from build123d import *

# Parameters (mm, degrees)
BOSS_EXTRUDE1_DEPTH = 9
SKETCH2_R           = 2.5
CUT_EXTRUDE1_DEPTH  = 39.913365313
BOSS_EXTRUDE2_DEPTH = 4.5
CUT_EXTRUDE2_DEPTH  = 3.5


with BuildPart() as part:
    # Sketch1 → Boss-Extrude1 (new body)
    with BuildSketch(Plane.XY):
        with BuildLine():
            Line((0, 0), (0, -5.580710666))
            ThreePointArc((0, -5.580710666), (0.901780583, -8.110737631), (3.200518222, -9.5))
            Line((3.200518222, -9.5), (13.019339267, -11.502906099))
            ThreePointArc((13.019339267, -11.502906099), (17.074073947, -15.986411077), (14, -21.191481642))
            Line((14, -21.191481642), (14, -31.5))
            Line((14, -31.5), (21, -31.5))
            Line((21, -31.5), (21, -5.5))
            Line((21, -5.5), (4, -5.5))
            Line((4, -5.5), (4, 0))
            Line((4, 0), (0, 0))
        make_face()
    extrude(amount=BOSS_EXTRUDE1_DEPTH)

    # Sketch2 → Cut-Extrude1 (cut, through all)
    with BuildSketch(Plane(origin=(21, 0, 0), x_dir=(0, 0, -1), z_dir=(1, 0, 0))):
        with Locations((-6, -25.5)):
            Circle(SKETCH2_R)
    extrude(amount=-CUT_EXTRUDE1_DEPTH, mode=Mode.SUBTRACT)

    # Sketch3 → Boss-Extrude2 (add)
    with BuildSketch(Plane.XY.offset(9)):
        with BuildLine():
            Line((12, -5.5), (12, -11.294974737))
            Line((12, -11.294974737), (13.019339267, -11.502906099))
            ThreePointArc((13.019339267, -11.502906099), (17.074073947, -15.986411077), (14, -21.191481642))
            Line((14, -21.191481642), (14, -31.5))
            Line((14, -31.5), (21, -31.5))
            Line((21, -31.5), (21, -5.5))
            Line((21, -5.5), (12, -5.5))
        make_face()
    extrude(amount=BOSS_EXTRUDE2_DEPTH)

    # Sketch4 → Cut-Extrude2 (cut)
    with BuildSketch(Plane(origin=(21, 0, 0), x_dir=(0, 0, -1), z_dir=(1, 0, 0))):
        Polygon((-10.2, -23.652479139), (-10.2, -27.347520861), (-6, -29.772391992), (-2.3, -27.636195996), (-2.3, -23.363804004), (-6, -21.227608008), align=None)
    extrude(amount=-CUT_EXTRUDE2_DEPTH, mode=Mode.SUBTRACT)


solid = part.part
Check sheet for the modelled part. Datum: model origin and axes. Units: mm. A direction names the side the tool comes from. Give positions to 0.01 mm unless a question says otherwise; leave off trailing zeros. Loops run counter-clockwise (first coordinate to the right, second up) from the corner with the lowest first, then second, coordinate; pieces in that order, holes last. Notation, with made-up numbers: M 27,11 L 44,11 A6 cw 44,17 Z; hole C 67.5,14.5 d3. An arc over 180 degrees is marked long. Use a Markdown table: item, result. Add a question column.
Q1. Sectioned sample at B-B, the plane x = 15. Record the cut outline in (y, z).
Q2. Scan lines: line 1 along Y through (x, z) = (15.1, 6); line 2 along X through (y, z) = (-28, 1.75); line 3 along X through (y, z) = (-10, 11). Record each from-to range of solid material in increasing order. Write a range as [from, to].
Q3. Sectioned sample at A-A, the plane y = -25.5. Record the cut outline in (x, z).
Q4. Mould release check, pull along Y, two halves, no side actions. Record for faces 5 (the flat face through (17.5, -23.5, 8.1)), 6 (the flat face through (6, -7, 9)), 7 (the flat face through (19.274, -22.423, 8.071)), 8 (the flat face through (17, -31.5, 7)): pulls with the +Y half, pulls with the -Y half, needs draft (parallel to the pull), parting line crosses it, or undercut.
Q5. Sectioned sample at D-D, the plane x = 18.75. Record the cut outline in (y, z), then the cut area to 3 significant figures.
Q6. Sectioned sample at C-C, the plane z = 12.5. Record the cut outline in (x, y).
Q7. Tool access check on faces 1 (the flat face through (19.27, -28.72, 4.18)), 2 (the flat face through (14, -27.4, 8.2)), 3 (the flat face through (12, -8, 11)), 4 (the flat face through (4, -3, 4)). Record the directions out of +Z, -Z, +X, -X, +Y, -Y that give a thin tool (end or side, any length) a straight path to the whole face; none if there is none.
Q8. Go/stop test with flat-tipped pins: pin 1 (2 mm diameter, centred on x = 9.5, z = 2.5, fed in from -Y); pin 2 (12 mm diameter, centred on x = 8, y = -18.5, fed in from +Z); pin 3 (3 mm diameter, centred on x = 14.5, z = 5.5, fed in from +Y); pin 4 (6 mm diameter, centred on y = -25.5, z = 6, fed in from +X). Record where each tip stops, or that it passes through.
Verdict:
| question | item | result |
|---|---|---|
| 1 | outline | M -31.5,0 L -20.62,0 L -20.62,13.5 L -31.5,13.5 Z; M -12.38,0 L -5.5,0 L -5.5,13.5 L -12.38,13.5 Z; hole C -25.5,6 d5 |
| 2 | line 1 | [-31.5, -28], [-23, -20.55], [-12.45, -5.5] |
| 2 | line 2 | [14, 21] |
| 2 | line 3 | [12, 21] |
| 3 | outline | M 14,0 L 21,0 L 21,2.3 L 17.5,2.3 L 17.5,3.5 L 14,3.5 Z; M 14,8.5 L 17.5,8.5 L 17.5,10.2 L 21,10.2 L 21,13.5 L 14,13.5 Z |
| 4 | face 5 | undercut |
| 4 | face 6 | needs draft |
| 4 | face 7 | undercut |
| 4 | face 8 | pulls with the -Y half |
| 5 | outline | M -31.5,0 L -5.5,0 L -5.5,13.5 L -31.5,13.5 Z; hole M -29.77,6 L -27.64,2.3 L -23.36,2.3 L -21.23,6 L -23.65,10.2 L -27.35,10.2 Z |
| 5 | area | 302 mm^2 |
| 6 | outline | M 12,-11.29 L 13.02,-11.5 A5.1 cw 14,-21.19 L 14,-31.5 L 21,-31.5 L 21,-5.5 L 12,-5.5 Z |
| 7 | face 1 | +X |
| 7 | face 2 | +Z, -Z, -X, -Y |
| 7 | face 3 | +Z, -X, +Y, -Y |
| 7 | face 4 | +Z, -Z, +X, +Y |
| 8 | pin 1 | y = -10.99 |
| 8 | pin 2 | through |
| 8 | pin 3 | y = -5.5 |
| 8 | pin 4 | x = 17.5 |
